Check sheet for the modelled part. Datum: model origin and axes. Units: mm. A direction names the side the tool comes from. Give positions to 0.01 mm unless a question says otherwise; leave off trailing zeros.
from build123d import *

# Parameters (mm, degrees)
BOX007_W               = 100
BOX007_H               = 100
BOX007_DEPTH           = 100
BOX007_PLACEMENT_ANGLE = 45
BOX006_W               = 200
BOX006_H               = 100
BOX006_DEPTH           = 100
BOX006_PLACEMENT_ANGLE = 45
BOX005_W               = 100
BOX005_H               = 100
BOX005_DEPTH           = 100
BOX005_PLACEMENT_ANGLE = -90
BOX004_W               = 20
BOX004_H               = 20
BOX004_DEPTH           = 80
BOX003_W               = 20
BOX003_H               = 20
BOX003_DEPTH           = 80
BOX002_W               = 10
BOX002_H               = 25
BOX002_DEPTH           = 35
BOX002_PITCH_ANGLE     = -15
BOX001_W               = 10
BOX001_H               = 25
BOX001_DEPTH           = 35
BOX001_PITCH_ANGLE     = 15
BOX_W                  = 20
BOX_H                  = 25
BOX_DEPTH              = 35
CYLINDER005_R          = 10
CYLINDER005_DEPTH      = 180
CYLINDER005_ROLL_ANGLE = 90
CYLINDER004_R          = 54
CYLINDER004_DEPTH      = 100
CYLINDER003_R          = 59
CYLINDER003_DEPTH      = 10
CYLINDER002_R          = 64
CYLINDER002_DEPTH      = 85
CYLINDER001_R          = 70
CYLINDER001_DEPTH      = 90
CYLINDER_R             = 80
CYLINDER_DEPTH         = 10
FILLET_R               = 3
FILLET001_R            = 5
FILLET002_R            = 5
CUT009_ROLL_ANGLE      = -90
CUT009_PITCH_ANGLE     = -45
CUT009_PLACEMENT_ANGLE = 45


with BuildPart() as cube004:
    # Box007 → Box007 (new body)
    with BuildSketch(Plane.XY):
        with Locations((50, 50)):
            Rectangle(BOX007_W, BOX007_H)
    extrude(amount=BOX007_DEPTH)


with BuildPart() as cube004_1:
    # Box007 placement: moved
    add(cube004.part.rotate(Axis((0, 0, 0), (0, 0, 1)), BOX007_PLACEMENT_ANGLE))


with BuildPart() as cube003:
    # Box006 → Box006 (new body)
    with BuildSketch(Plane.XY):
        with Locations((100, 50)):
            Rectangle(BOX006_W, BOX006_H)
    extrude(amount=BOX006_DEPTH)


with BuildPart() as cube003_1:
    # Box006 placement: moved
    add(cube003.part.moved(Location((-71, -71, 0))).rotate(Axis((-71, -71, 0), (0, 0, 1)), BOX006_PLACEMENT_ANGLE))


with BuildPart() as cube002:
    # Box005 → Box005 (new body)
    with BuildSketch(Plane.XY):
        with Locations((50, 50)):
            Rectangle(BOX005_W, BOX005_H)
    extrude(amount=BOX005_DEPTH)


with BuildPart() as cube002_1:
    # Box005 placement: moved
    add(cube002.part.rotate(Axis((0, 0, 0), (0, 0, 1)), BOX005_PLACEMENT_ANGLE))


with BuildPart() as tab_cut_l:
    # Box004 → Box004 (new body)
    with BuildSketch(Plane(origin=(-83, -10, 20), x_dir=(1, 0, 0), z_dir=(0, 0, 1))):
        with Locations((10, 10)):
            Rectangle(BOX004_W, BOX004_H)
    extrude(amount=BOX004_DEPTH)


with BuildPart() as tab_cut_r:
    # Box003 → Box003 (new body)
    with BuildSketch(Plane(origin=(63, -10, 20), x_dir=(1, 0, 0), z_dir=(0, 0, 1))):
        with Locations((10, 10)):
            Rectangle(BOX003_W, BOX003_H)
    extrude(amount=BOX003_DEPTH)


with BuildPart() as cube001:
    # Box002 → Box002 (new body)
    with BuildSketch(Plane.XY):
        with Locations((5, 12.5)):
            Rectangle(BOX002_W, BOX002_H)
    extrude(amount=BOX002_DEPTH)


with BuildPart() as cube001_1:
    # Box002 pitch: moved
    add(cube001.part.rotate(Axis((0, 0, 0), (0, 1, 0)), BOX002_PITCH_ANGLE))


with BuildPart() as cube001_2:
    # Box002 placement: moved
    add(cube001_1.part.moved(Location((-9.95, 48, 64))))


with BuildPart() as cube:
    # Box001 → Box001 (new body)
    with BuildSketch(Plane.XY):
        with Locations((5, 12.5)):
            Rectangle(BOX001_W, BOX001_H)
    extrude(amount=BOX001_DEPTH)


with BuildPart() as cube_1:
    # Box001 pitch: moved
    add(cube.part.rotate(Axis((0, 0, 0), (0, 1, 0)), BOX001_PITCH_ANGLE))


with BuildPart() as cube_2:
    # Box001 placement: moved
    add(cube_1.part.moved(Location((0, 48, 65))))


with BuildPart() as bearing_slot:
    # Box → Box (new body)
    with BuildSketch(Plane(origin=(-10, 48, 65), x_dir=(1, 0, 0), z_dir=(0, 0, 1))):
        with Locations((10, 12.5)):
            Rectangle(BOX_W, BOX_H)
    extrude(amount=BOX_DEPTH)


with BuildPart() as bearing_holes:
    # Cylinder005 → Cylinder005 (new body)
    with BuildSketch(Plane.XY):
        Circle(CYLINDER005_R)
    extrude(amount=CYLINDER005_DEPTH)


with BuildPart() as bearing_holes_1:
    # Cylinder005 roll: moved
    add(bearing_holes.part.rotate(Axis((0, 0, 0), (1, 0, 0)), CYLINDER005_ROLL_ANGLE))


with BuildPart() as bearing_holes_2:
    # Cylinder005 placement: moved
    add(bearing_holes_1.part.moved(Location((0, 90, 65))))


with BuildPart() as through_hole:
    # Cylinder004 → Cylinder004 (new body)
    with BuildSketch(Plane.XY):
        Circle(CYLINDER004_R)
    extrude(amount=CYLINDER004_DEPTH)


with BuildPart() as inner_lip:
    # Cylinder003 → Cylinder003 (new body)
    with BuildSketch(Plane.XY.offset(80)):
        Circle(CYLINDER003_R)
    extrude(amount=CYLINDER003_DEPTH)


with BuildPart() as inner_hole:
    # Cylinder002 → Cylinder002 (new body)
    with BuildSketch(Plane.XY):
        Circle(CYLINDER002_R)
    extrude(amount=CYLINDER002_DEPTH)


with BuildPart() as body_cylinder:
    # Cylinder001 → Cylinder001 (new body)
    with BuildSketch(Plane.XY.offset(5)):
        Circle(CYLINDER001_R)
    extrude(amount=CYLINDER001_DEPTH)


with BuildPart() as cut010:
    # Cylinder → Cylinder (new body)
    with BuildSketch(Plane.XY):
        Circle(CYLINDER_R)
    extrude(amount=CYLINDER_DEPTH)

    # Fusion: union Body_Cylinder
    add(body_cylinder.part)

    # Cut: cut Inner_Hole
    add(inner_hole.part, mode=Mode.SUBTRACT)

    # Fusion001: union Inner_Lip
    add(inner_lip.part)

    # Cut001: cut Through_Hole
    add(through_hole.part, mode=Mode.SUBTRACT)

    # Fillet
    fillet_edges = [cut010.edges().sort_by_distance(p)[0] for p in [
        (-70, 0, 10),
    ]]
    fillet(fillet_edges, radius=FILLET_R)

    # Fillet001
    fillet001_edges = [cut010.edges().sort_by_distance(p)[0] for p in [
        (-80, 0, 0),
    ]]
    fillet(fillet001_edges, radius=FILLET001_R)

    # Fillet002
    fillet002_edges = [cut010.edges().sort_by_distance(p)[0] for p in [
        (-70, 0, 95),
    ]]
    fillet(fillet002_edges, radius=FILLET002_R)

    # Cut002: cut Bearing_Holes
    add(bearing_holes_2.part, mode=Mode.SUBTRACT)

    # Cut003: cut Bearing_Slot
    add(bearing_slot.part, mode=Mode.SUBTRACT)

    # Cut004: cut Cube
    add(cube_2.part, mode=Mode.SUBTRACT)

    # Cut005: cut Cube001
    add(cube001_2.part, mode=Mode.SUBTRACT)

    # Cut006: cut Tab_Cut_R
    add(tab_cut_r.part, mode=Mode.SUBTRACT)

    # Cut007: cut Tab_Cut_L
    add(tab_cut_l.part, mode=Mode.SUBTRACT)

    # Cut008: cut Cube002
    add(cube002_1.part, mode=Mode.SUBTRACT)

    # Cut009: cut Cube003
    add(cube003_1.part, mode=Mode.SUBTRACT)


with BuildPart() as cut010_1:
    # Cut009 roll: moved
    add(cut010.part.rotate(Axis((0, 0, 0), (1, 0, 0)), CUT009_ROLL_ANGLE))


with BuildPart() as cut010_2:
    # Cut009 pitch: moved
    add(cut010_1.part.rotate(Axis((0, 0, 0), (0, 1, 0)), CUT009_PITCH_ANGLE))


with BuildPart() as cut010_3:
    # Cut009 placement: moved
    add(cut010_2.part.rotate(Axis((0, 0, 0), (0, 0, 1)), CUT009_PLACEMENT_ANGLE))

    # Cut010: cut Cube004
    add(cube004_1.part, mode=Mode.SUBTRACT)


solid = cut010_3.part
1) Draft check along X on faces 1 (the flat face through (-92.861, 20.276, 21.687)), 2 (the flat face through (-99.11, 21.1, 23.02)), 3 (the cylindrical face through (-81.87, -9.8, 26.43)). Enter one of: +X half, -X half, draft (parallel to the pull), parting line (faces both ways), or undercut.
2) Scan lines: L1, parallel to Y at x = -103.5, z = 7; L2, parallel to X at y = -24.5, z = 13; L3, parallel to Z at x = -67, y = 2. Record each from-to range of solid material in increasing order.
3) Gauge pin test, flat ends, axial feed: pin 1 (3 mm diameter, centred on y = -36.5, z = 29, fed in from -X); pin 2 (6 mm diameter, centred on x = -68, y = -15.5, fed in from +Z); pin 3 (1 mm diameter, centred on y = -23.5, z = 19.5, fed in from +X). Record the tip position at first contact, or that the pin passes through.
4) Access from +Z, -Z, +X, -X, +Y, -Y to the whole of each face (thin tool, end or side, straight path). Record for faces 4 (the cylindrical face through (-96.94, 19.68, 22.28)), 5 (the flat face through (-56.25, -42.11, 29.37)), 6 (the cylindrical face through (-57.66, -47.1, 30.21)).
Answers below:
1. face 1: +X half
1. face 2: undercut
1. face 3: -X half
2. L1: y = 5 to 13.53, 16.71 to 27.78
2. L2: x = -72.77 to -64.12
2. L3: z = 44.54 to 45.96
3. pin 1: stops at x = -55.38
3. pin 2: stops at z = 41.94
3. pin 3: stops at x = -62.16
4. face 4: none
4. face 5: +Z, -X
4. face 6: +Z, -X, -Y
